For this review, take the finished solid that the model builds, in its own axes (mm). A direction names the side the tool comes from. Give positions to 0.01 mm unless a question says otherwise; leave off trailing zeros. Loops run counter-clockwise (first coordinate to the right, second up) from the corner with the lowest first, then second, coordinate; pieces in that order, holes last. Notation, with made-up numbers: (-7.5, -6.75) -> (37.5, -6.75) arc R27 cw to (37.5, 22.25) -> close; hole circle Ø9 at (85, 57). An arc over 180 degrees is marked (long way). One line per question, with ' | ' between items. Start each with the question number.
(1) Draft analysis for pull direction Y (two halves, no side actions). For faces 1 (the flat face through (-223, 119.455, 1280)), 2 (the flat face through (-190.046, 87, 1280)), 3 (the cylindrical face through (-195.102, 57.756, 1273.588)), state which applies: +Y half, -Y half, draft (parallel to the pull), parting line (faces both ways), or undercut.
(2) Tool access review of faces 4 (the flat face through (-249, 86, 1265.776)), 5 (the flat face through (-212, 66.901, 1280)), 6 (the cylindrical face through (-254.08, 85.52, 1272.11)): name each direction out of +Z, -Z, +X, -X, +Y, -Y from which nothing blocks a thin tool from reaching the whole face with its end or side.
(3) Consider section A-A (x = -207). Write out the cut boundary in (y, z).
(4) Consider section C-C (z = 1273.25). Write out the cut boundary in (x, y), and give its area (3 significant figures).
(5) Consider section B-B (y = 96). Write out the cut boundary in (x, z), and give its area (3 significant figures).
(6) Consider section D-D (x = -239.5). Write out the cut boundary in (y, z).
(7) Insertion check: P1, Ø3.5, axis at x = -194.05, y = 115.45, coming from the +Z side; P2, Ø8, axis at x = -239.5, y = 72.5, coming from the -Z side. Each pin has a flat end and moves straight along its axis. Give the tip position at first contact, or say it passes through.
(8) Wall thickness on probe 1 along Y at (x, z) = (-251, 1276.75); probe 2 along Z at (x, y) = (-196.5, 70); probe 3 along Y at (x, z) = (-193.5, 1280.75): over which ranges is each line inside the solid? List them lowest first.
from build123d import *

# Parameters (mm, degrees)
SKETCH1_W             = 65
SKETCH1_H             = 64
BOSS_EXTRUDE1_DEPTH   = 3
F_4_0MM_DOWEL_HOLE1_D = 4
BOSS_EXTRUDE2_START   = 12.845580916
SKETCH4_R             = 3.6
SKETCH4_R_2           = 2
BOSS_EXTRUDE2_DEPTH   = 12.845580916
CUT_EXTRUDE4_REACH    = 284.08
SKETCH5_W             = 30
SKETCH5_H             = 31


with BuildPart() as part:
    # Sketch1 → Boss-Extrude1 (new body)
    with BuildSketch(Plane(origin=(0, -5.589e-05, 1278.621377902), x_dir=(1, 0, 0), z_dir=(0, -4.371138800000001e-08, 0.999999999999999))):
        with Locations((-222.546248068, 87.454866132)):
            Rectangle(SKETCH1_W, SKETCH1_H)
    extrude(amount=BOSS_EXTRUDE1_DEPTH)

    # Ø4.0mm Dowel Hole1 (through all)
    with Locations(Plane(origin=(0, -5.6021e-05, 1281.621377902), x_dir=(-1, 0, 0), z_dir=(0, -4.371138867531602e-08, 0.999999999999999))):
        with Locations((251.046248068, -87.454866132), (194.046248068, -115.454866132), (194.046248068, -59.454866132)):
            Hole(F_4_0MM_DOWEL_HOLE1_D / 2)

    # Sketch4 → Boss-Extrude2 (add)
    # profile 1 of 3: a face of its own
    with BuildSketch(Plane(origin=(0, -5.589e-05, 1278.621377902), x_dir=(-1, 0, 0), z_dir=(0, 4.371138867531603e-08, -0.9999999999999991)).offset(BOSS_EXTRUDE2_START)):
        with Locations(Location((194.046248068, 115.454866132, 0), (0, 0, 270))):
            Circle(SKETCH4_R)
        with Locations(Location((194.046248068, 115.454866132, 0), (0, 0, 270))):
            Circle(SKETCH4_R_2, mode=Mode.SUBTRACT)
    # profile 2 of 3: a face of its own
    with BuildSketch(Plane(origin=(0, -5.589e-05, 1278.621377902), x_dir=(-1, 0, 0), z_dir=(0, 4.371138867531603e-08, -0.9999999999999991)).offset(BOSS_EXTRUDE2_START)):
        with Locations(Location((251.046248068, 87.454866132, 0), (0, 0, 270))):
            Circle(SKETCH4_R)
        with Locations(Location((251.046248068, 87.454866132, 0), (0, 0, 270))):
            Circle(SKETCH4_R_2, mode=Mode.SUBTRACT)
    # profile 3 of 3: a face of its own
    with BuildSketch(Plane(origin=(0, -5.589e-05, 1278.621377902), x_dir=(-1, 0, 0), z_dir=(0, 4.371138867531603e-08, -0.9999999999999991)).offset(BOSS_EXTRUDE2_START)):
        with Locations(Location((194.046248068, 59.454866132, 0), (0, 0, 270))):
            Circle(SKETCH4_R)
        with Locations(Location((194.046248068, 59.454866132, 0), (0, 0, 270))):
            Circle(SKETCH4_R_2, mode=Mode.SUBTRACT)
    extrude(amount=-BOSS_EXTRUDE2_DEPTH)

    # Sketch5 → Cut-Extrude4 (cut, up to next)
    with BuildSketch(Plane(origin=(0, -5.6021e-05, 1281.621377902), x_dir=(1, 0, 0), z_dir=(0, -4.371138867531602e-08, 0.999999999999999)), mode=Mode.PRIVATE) as cut_extrude4_sk1:
        with Locations((-212.038243782, 82.401305574)):
            Rectangle(SKETCH5_W, SKETCH5_H)
    cut_extrude4_tool1 = extrude(cut_extrude4_sk1.sketch, amount=-CUT_EXTRUDE4_REACH, mode=Mode.PRIVATE) & part.part
    add(cut_extrude4_tool1.solids().sort_by_distance((-212.038244, 82.40125, 1281.621382))[0], mode=Mode.SUBTRACT)


solid = part.part
A:
1) face 1: +Y half | face 2: draft | face 3: undercut
2) face 4: -Z, +X, -X, +Y, -Y | face 5: +Z, -Z | face 6: -Z
3) outline: (55.45, 1278.62) -> (66.9, 1278.62) -> (66.9, 1281.62) -> (55.45, 1281.62) -> close; (97.9, 1278.62) -> (119.45, 1278.62) -> (119.45, 1281.62) -> (97.9, 1281.62) -> close
4) outline: circle Ø7.2 at (-251.05, 87.45); circle Ø7.2 at (-194.05, 59.45); circle Ø7.2 at (-194.05, 115.45); hole circle Ø4 at (-251.05, 87.45); hole circle Ø4 at (-194.05, 59.45); hole circle Ø4 at (-194.05, 115.45) | area: 84.4 mm^2
5) outline: (-255.05, 1278.62) -> (-227.04, 1278.62) -> (-227.04, 1281.62) -> (-255.05, 1281.62) -> close; (-197.04, 1278.62) -> (-190.05, 1278.62) -> (-190.05, 1281.62) -> (-197.04, 1281.62) -> close | area: 105 mm^2
6) outline: (55.45, 1278.62) -> (119.45, 1278.62) -> (119.45, 1281.62) -> (55.45, 1281.62) -> close
7) P1: passes through | P2: stops at z = 1278.62
8) probe 1: y = 83.86 to 85.46, 89.45 to 91.05 | probe 2: z = 1278.62 to 1281.62 | probe 3: y = 55.45 to 57.53, 61.38 to 113.53, 117.38 to 119.45
